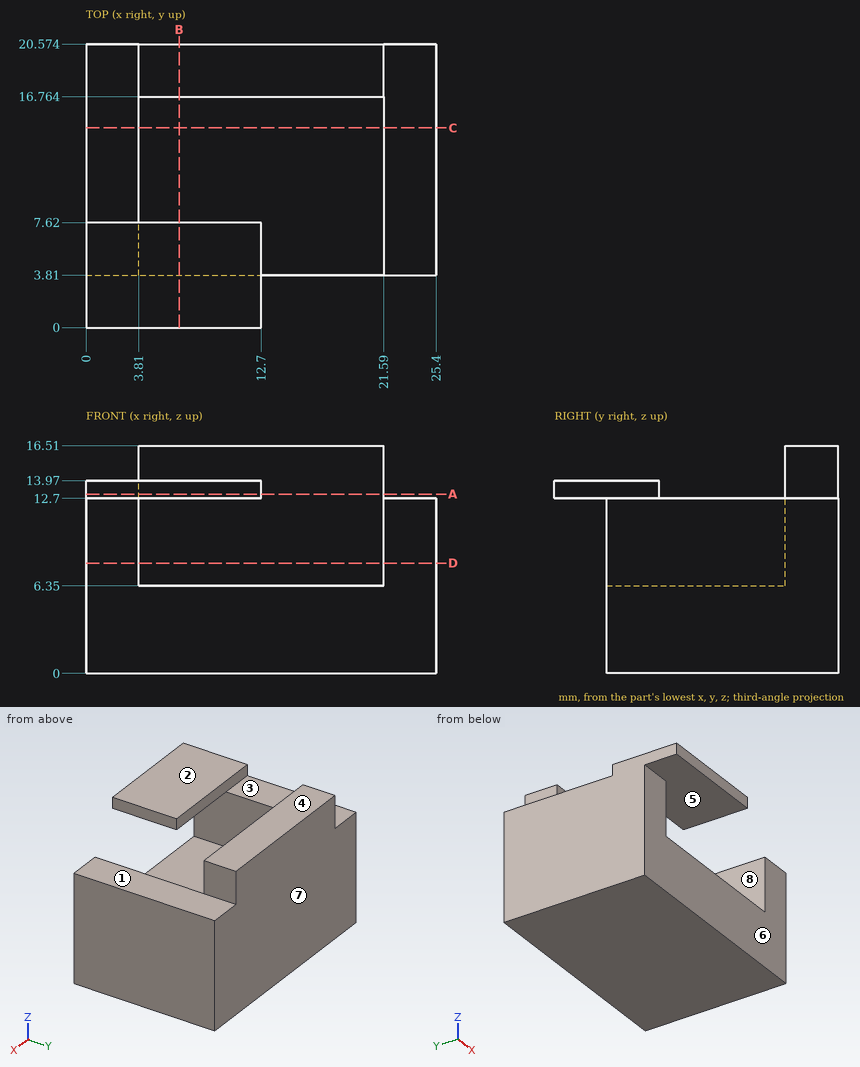
Verification items for this drawing (mm, ordinates from the low corner). A direction names the side the tool comes from. Give positions to 0.01 mm unless a question says otherwise; leave off trailing zeros. Write each loop counter-clockwise with the first axis right and the second up, starting at its lowest first coordinate (ties: lowest second). Pieces come first, ordered by that corner, then holes.
1) Section check D-D, the plane z = 8. Record the boundary of the cut face in (x, y).
2) Release check for a two-part mould opening along Y. For the marked faces 6, 7 and 8 record: pulls with the +Y half, pulls with the -Y half, needs draft (parallel to the pull), parting line crosses it, or undercut.
3) Gauge pin test, flat ends, axial feed: pin 1 (2.5 mm diameter, centred on x = 9, y = 5.5, fed in from +Z); pin 2 (1.9 mm diameter, centred on x = 23, y = 13, fed in from +Z); pin 3 (1.9 mm diameter, centred on y = 9, z = 10, fed in from -X); pin 4 (1.9 mm diameter, centred on y = 18.5, z = 15.5, fed in from +X). Record the tip position at first contact, or that the pin passes through.
4) Access from +Z, -Z, +X, -X, +Y, -Y to the whole of each face (thin tool, end or side, straight path). Record for the marked faces 1, 2, 3, 4 and 5.
5) Section check B-B, the plane x = 6.75. Record the boundary of the cut face in (y, z), and give its area (3 significant figures).
6) Section check A-A, the plane z = 13. Record the boundary of the cut face in (x, y), and give its area (3 significant figures).
7) Material ranges on L1, parallel to Z at x = 9.5, y = 5.5; L2, parallel to X at y = 8, z = 10.75; L3, parallel to Z at x = 14, y = 16.25, recorded low to high.
8) Section check C-C, the plane y = 14.5. Record the boundary of the cut face in (x, z).
Computed:
1. outline: (0, 3.81) - (3.81, 3.81) - (3.81, 16.76) - (21.59, 16.76) - (21.59, 3.81) - (25.4, 3.81) - (25.4, 20.57) - (0, 20.57) - close
2. face 6: pulls with the -Y half
2. face 7: pulls with the +Y half
2. face 8: needs draft
3. pin 1: stops at z = 13.97
3. pin 2: stops at z = 12.7
3. pin 3: stops at x = 0
3. pin 4: stops at x = 21.59
4. face 1: +Z, +X, +Y, -Y
4. face 2: +Z, +X, -X, -Y
4. face 3: +Z, -X, +Y
4. face 4: +Z, +X, -X, +Y, -Y
4. face 5: -Y
5. outline: (0, 12.7) - (7.62, 12.7) - (7.62, 13.97) - (0, 13.97) - close; (3.81, 0) - (20.57, 0) - (20.57, 16.51) - (16.76, 16.51) - (16.76, 6.35) - (3.81, 6.35) - close
5. area: 155 mm2
6. outline: (0, 0) - (12.7, 0) - (12.7, 7.62) - (0, 7.62) - close; (3.81, 16.76) - (21.59, 16.76) - (21.59, 20.57) - (3.81, 20.57) - close
6. area: 165 mm2
7. L1: z = 0 to 6.35, 12.7 to 13.97
7. L2: x = 0 to 3.81, 21.59 to 25.4
7. L3: z = 0 to 6.35
8. outline: (0, 0) - (25.4, 0) - (25.4, 12.7) - (21.59, 12.7) - (21.59, 6.35) - (3.81, 6.35) - (3.81, 12.7) - (0, 12.7) - close
